Work out the finished part from the listing and answer in its coordinate system (mm). Give positions to 0.01 mm unless a question says otherwise; leave off trailing zeros. Loops run counter-clockwise (first coordinate to the right, second up) from the corner with the lowest first, then second, coordinate; pieces in that order, holes last. Notation, with made-up numbers: M 71,-23 L 116,-23 A21 cw 116,-1 Z; hole C 78.5,-7 d10. An arc over 180 degrees is marked long. Use a Markdown table: item, result.
```python
from build123d import *

# Parameters (mm, degrees)
SKETCH1_W            = 140
SKETCH1_H            = 140
BOSS_EXTRUDE1_DEPTH  = 10
M4_CLEARANCE_HOLE1_D = 4.5


with BuildPart() as part:
    # Sketch1 → Boss-Extrude1 (new body)
    with BuildSketch(Plane(origin=(0, 0, 0), x_dir=(1, 0, 0), z_dir=(0, 1, 0))):
        Rectangle(SKETCH1_W, SKETCH1_H)
    extrude(amount=-BOSS_EXTRUDE1_DEPTH)

    # M4 Clearance Hole1 (through all)
    with Locations(Plane(origin=(0, 0, 0), x_dir=(1, 0, 0), z_dir=(0, 1, 0))):
        with Locations((-45, 45), (-45, -45), (45, -45), (45, 45), (25, 25), (-25, 25), (-25, -25), (25, -25)):
            Hole(M4_CLEARANCE_HOLE1_D / 2)


solid = part.part
```
(1) A cutting plane is placed at B-B (z = 25). Write down the section's boundary in (x, y).
Entries:
| item | result |
|---|---|
| outline | M -70,-10 L -27.25,-10 L -27.25,0 L -70,0 Z; M -22.75,-10 L 22.75,-10 L 22.75,0 L -22.75,0 Z; M 27.25,-10 L 70,-10 L 70,0 L 27.25,0 Z |
(2) Given P1, Ø5, axis at x = -45, z = -45, coming from the -Y side, flat-ended and moving along its own axis, determine where the tip first touches the part or whether it passes through.
Entries:
| item | result |
|---|---|
| P1 | stops at y = -10 |
(3) Consider probe 1 along Z at (x, y) = (-45, -7.25); probe 2 along Z at (x, y) = (-25, -7.25). Determine where each line is inside the solid, lowest interval first. Write a range as [from, to].
Entries:
| item | result |
|---|---|
| probe 1 | z = [-70, -47.25], [-42.75, 42.75], [47.25, 70] |
| probe 2 | z = [-70, -27.25], [-22.75, 22.75], [27.25, 70] |
(4) The mould has two halves that part along Z. Classify faces 1 (the cylindrical face through (-43.34, -5.07, 43.48)), 2 (the flat face through (70, -5, 1)), 3 (the cylindrical face through (-26.038, -5.07, -23.004)), 4 (the flat face through (-1, -5, -70)): released by +Z, released by -Z, zero draft, split by the parting line, or undercut.
Entries:
| item | result |
|---|---|
| face 1 | undercut |
| face 2 | zero draft |
| face 3 | undercut |
| face 4 | released by -Z |
(5) A cutting plane is placed at A-A (x = -45). Write down the section's boundary in (y, z).
Entries:
| item | result |
|---|---|
| outline | M -10,-70 L 0,-70 L 0,-47.25 L -10,-47.25 Z; M -10,-42.75 L 0,-42.75 L 0,42.75 L -10,42.75 Z; M -10,47.25 L 0,47.25 L 0,70 L -10,70 Z |
